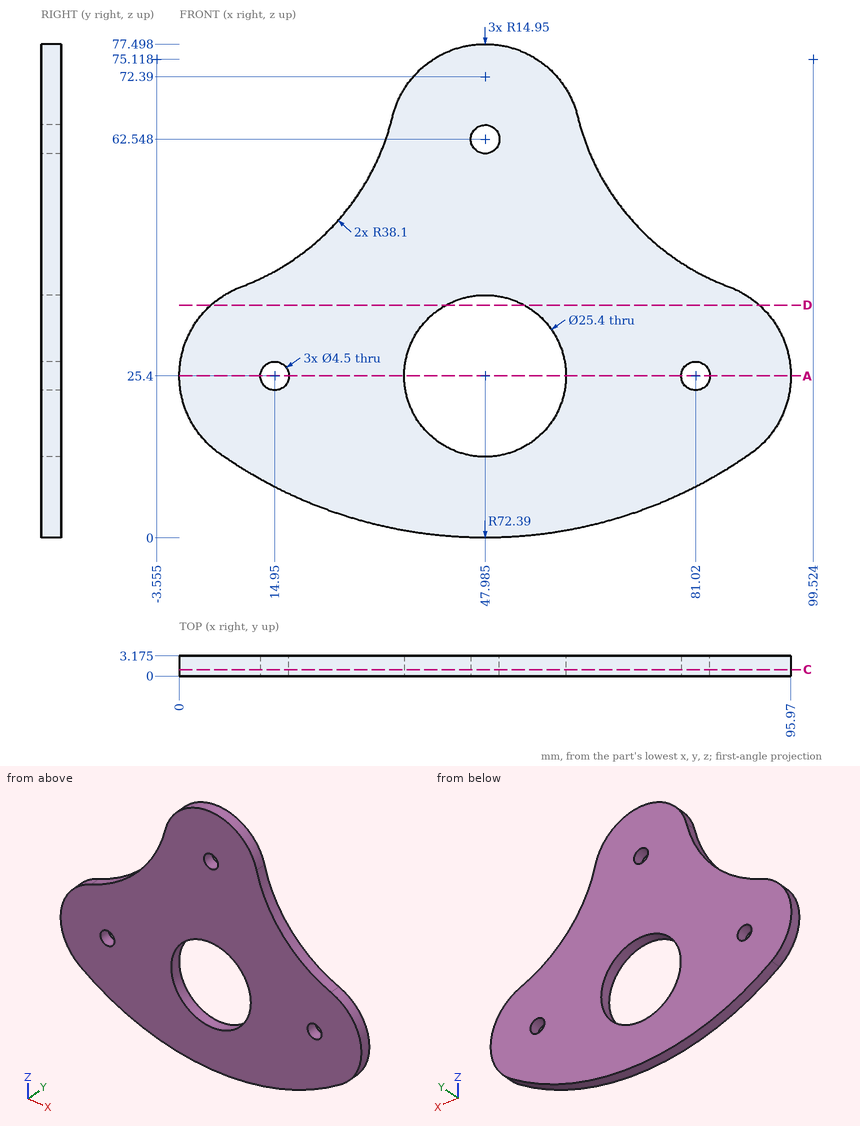
For this review, use the dimensioned drawing (mm, ordinates from the lowest corner) and the shaded views. Round coordinates to 2 decimals unless told otherwise and drop trailing zeros. Order: outer loops, then holes, each group sorted by start corner. A loop starts at its lowest first (then second) coordinate and runs counter-clockwise, first axis right, second up. Notation, with made-up numbers: (66, 81) -> (103, 81) arc R23 ccw to (103, 105) -> close; hole circle Ø6 at (1, -22.5). An arc over 180 degrees is marked (long way). Use CSV: the item, a comma, the result in double quotes. Start each with the question number.
(1) Wall thickness on probe 1 along X at (y, z) = (2.55, 25.4) (1 decimal); probe 2 along Z at (x, y) = (16.5, 1.5) (1 decimal); probe 3 along Z at (x, y) = (37, 2.85) (1 decimal): over which ranges is each line inside the solid? List them lowest first. Write a range as from..to.
(2) Consider section D-D on z = 36.5. Write out the cut boundary in (x, y) (1 decimal).
(3) Insertion check: pin 1 (3.5 mm diameter, centred on x = 81.02, z = 25.4, fed in from -Y); pin 2 (10 mm diameter, centred on x = 19.5, z = 15.5, fed in from -Y). Each pin has a flat end and moves straight along its axis. Give the tip position at first contact, or say it passes through.
(4) Consider section A-A on z = 25.4. Write out the cut boundary in (x, y) (1 decimal).
(5) Consider section C-C on y = 1. State how many separate pieces and enclosed holes the cut face has, and give its area (3 significant figures).
Responses:
1,probe 1,"0..12.7, 17.2..35.3, 60.7..78.8, 83.3..96"
1,probe 2,"7.2..23.8, 27..42.7"
1,probe 3,"0.8..19, 31.8..72.7"
2,outline,"(4.9, 0) -> (41.8, 0) -> (41.8, 3.2) -> (4.9, 3.2) -> close; (54.2, 0) -> (91, 0) -> (91, 3.2) -> (54.2, 3.2) -> close"
3,pin 1,"through"
3,pin 2,"y = 0"
4,outline,"(0, 0) -> (12.7, 0) -> (12.7, 3.2) -> (0, 3.2) -> close; (17.2, 0) -> (35.3, 0) -> (35.3, 3.2) -> (17.2, 3.2) -> close; (60.7, 0) -> (78.8, 0) -> (78.8, 3.2) -> (60.7, 3.2) -> close; (83.3, 0) -> (96, 0) -> (96, 3.2) -> (83.3, 3.2) -> close"
5,separate pieces,"1"
5,enclosed holes,"4"
5,area,"4,030 mm²"
